```python
from build123d import *

# Parameters (mm, degrees)
ODGI_CIE_BAZOWE1_DEPTH = 20
OTW_R_POD_RUB_M51_D    = 5.5
OTW_R_POD_RUB_M52_D    = 5.5
ZAOKR_GLENIE1_R        = 5


# Sheet-metal steps are written as plain solids
with BuildPart() as part:
    # Szkic1 → Odgięcie bazowe1 (new, symmetric)
    with BuildSketch(Plane(origin=(0, 0, 0), x_dir=(1, 0, 0), z_dir=(0, 1, 0))):
        with BuildLine():
            Line((0, -60), (0, -7))
            ThreePointArc((0, -7), (2.050252532, -2.050252532), (7, 0))
            Line((7, 0), (65, 0))
            Line((65, 0), (65, -3))
            Line((65, -3), (7, -3))
            ThreePointArc((7, -3), (4.171572875, -4.171572875), (3, -7))
            Line((3, -7), (3, -60))
            Line((3, -60), (0, -60))
        make_face()
    extrude(amount=ODGI_CIE_BAZOWE1_DEPTH, both=True)

    # Otwór pod śrubę M51 (through all)
    with Locations(Plane.XY.offset(3)):
        with Locations((27.5, 4), (40, -6), (52.5, 4)):
            Hole(OTW_R_POD_RUB_M51_D / 2)

    # Otwór pod śrubę M52 (through all)
    with Locations(Plane(origin=(3, 0, 0), x_dir=(0, 0, -1), z_dir=(1, 0, 0))):
        with Locations((-53, 12.5), (-33, 12.5), (-13, 12.5), (-13, -12.5), (-33, -12.5), (-53, -12.5)):
            Hole(OTW_R_POD_RUB_M52_D / 2)

    # Zaokrąglenie1
    zaokr_glenie1_edges = [part.edges().sort_by_distance(p)[0] for p in [
        (65, 20, 1.5),
        (65, -20, 1.5),
        (1.5, 20, 60),
        (1.5, -20, 60),
    ]]
    fillet(zaokr_glenie1_edges, radius=ZAOKR_GLENIE1_R)


solid = part.part
```
Geometry check sheet. Reference: the model listing, model coordinates, mm. A direction names the side the tool comes from. Coordinates: 2 decimals unless noted, no trailing zeros. Order: outer loops, then holes, each group sorted by start corner. A loop starts at its lowest first (then second) coordinate and runs counter-clockwise, first axis right, second up. Notation, with made-up numbers: M 89,-24.5 L 139,-24.5 A16 ccw 139,6.5 Z; hole C 52,-24.5 d1. An arc over 180 degrees is marked long. Answer as a JSON object with one key per item and string values.
Q1. Depth check by flat-ended pin: pin 1 Ø9 at (y, z) = (12.5, 13) entering from -X; pin 2 Ø7 at (x, y) = (27.5, 4) entering from +Z; pin 3 Ø6 at (y, z) = (6.5, 39.5) entering from +X; pin 4 Ø3.5 at (y, z) = (-12.5, 13) entering from -X. Enter the tip coordinate at first touch or a pass-through.
Results are:
{"pin 1": "stops at x = 0", "pin 2": "stops at z = 3", "pin 3": "stops at x = 3", "pin 4": "passes through"}
Q2. Cross-section at B-B on y = 12.5. Record the cut outline in (x, z), and give its area (3 significant figures).
Results are:
{"outline": "M 0,7 A7 ccw 7,0 L 65,0 L 65,3 L 7,3 A4 cw 3,7 L 3,10.25 L 0,10.25 Z; M 0,15.75 L 3,15.75 L 3,30.25 L 0,30.25 Z; M 0,35.75 L 3,35.75 L 3,50.25 L 0,50.25 Z; M 0,55.75 L 3,55.75 L 3,60 L 0,60 Z", "area": "309 mm²"}
Q3. Tool access check on faces 1 (the flat face through (3, 0, 33)), 2 (the cylindrical face through (42.747, -5.879, 1.479)). Record the directions out of +Z, -Z, +X, -X, +Y, -Y that give a thin tool (end or side, any length) a straight path to the whole face; none if there is none.
Results are:
{"face 1": "+Z, +X, +Y, -Y", "face 2": "+Z, -Z"}
Q4. Scan lines: line 1 (Y direction, x = 2, z = 53); line 2 (Y direction, x = 40, z = 1.6); line 3 (Y direction, x = 27.5, z = 1.75). Record each from-to range of solid material in increasing order.
Results are:
{"line 1": "y = -20 to -15.25, -9.75 to 9.75, 15.25 to 20", "line 2": "y = -20 to -8.75, -3.25 to 20", "line 3": "y = -20 to 1.25, 6.75 to 20"}
Q5. Cross-section at D-D on y = -1. Record the cut outline in (x, z).
Results are:
{"outline": "M 0,7 A7 ccw 7,0 L 65,0 L 65,3 L 7,3 A4 cw 3,7 L 3,60 L 0,60 Z"}
Q6. Cross-section at A-A on z = 53. Record the cut outline in (x, y), and give its area (3 significant figures).
Results are:
{"outline": "M 0,-20 L 3,-20 L 3,-15.25 L 0,-15.25 Z; M 0,-9.75 L 3,-9.75 L 3,9.75 L 0,9.75 Z; M 0,15.25 L 3,15.25 L 3,20 L 0,20 Z", "area": "87.0 mm²"}
Q7. Release check for a two-part mould opening along Z. For faces 3 (the cylindrical face through (2, 0.3, 2.1)), 4 (the cylindrical face through (1.479, -9.773, 12.642)), 5 (the cylindrical face through (1, -18, 59)), 6 (the cylindrical face through (63, -19, 2)) record: released by +Z, released by -Z, zero draft, split by the parting line, or undercut.
Results are:
{"face 3": "released by -Z", "face 4": "undercut", "face 5": "released by +Z", "face 6": "zero draft"}
Q8. Cross-section at C-C on x = 39. Record the cut outline in (y, z).
Results are:
{"outline": "M -20,0 L -8.56,0 L -8.56,3 L -20,3 Z; M -3.44,0 L 20,0 L 20,3 L -3.44,3 Z"}
